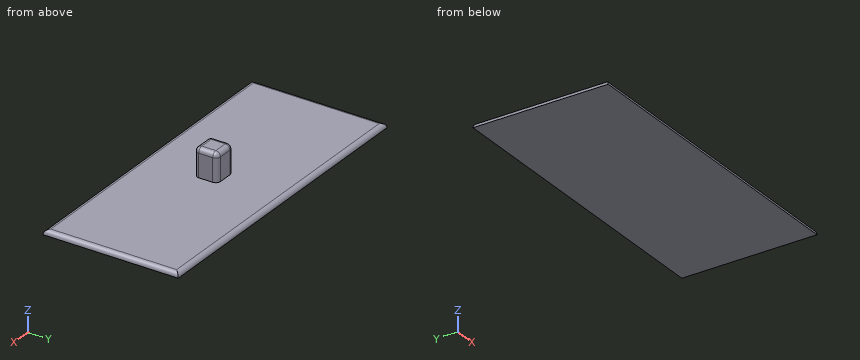
```python
from build123d import *

# Parameters (mm, degrees)
F0_W     = 170.18
F0_H     = 73.66
F1_DEPTH = 2.54
F2_W     = 12.7
F2_H     = 12.7
F3_DEPTH = 15.24
F4_R     = 2.53999


# Not quite as in the source:
# - a fillet or chamfer is up to 0.001 mm smaller than in the source, because OpenCascade refuses the exact size


with BuildPart() as f1:
    # F0 (on Top) → F1 (new body)
    with BuildSketch(Plane.XY):
        with Locations((1.0795005364, 0)):
            Rectangle(F0_W, F0_H)
    extrude(amount=F1_DEPTH)

    # F2 (on face) → F3 (join)
    with BuildSketch(Plane.XY.offset(2.54)):
        with Locations((0, -1.5238544315)):
            Rectangle(F2_W, F2_H)
    extrude(amount=F3_DEPTH)

    # F4 (radius 2.54 in the source; OpenCascade refuses exactly that, so slightly less here)
    f4_edges = [f1.edges().sort_by_distance(p)[0] for p in [
        (0, -7.873854, 17.78),
        (-6.35, -1.523854, 17.78),
        (0, 4.826146, 17.78),
        (6.35, -1.523854, 17.78),
        (-6.35, -7.873854, 10.16),
        (6.35, -7.873854, 10.16),
        (6.35, 4.826146, 10.16),
        (-6.35, 4.826146, 10.16),
        (1.079501, -36.83, 2.54),
        (86.169501, 0, 2.54),
        (1.079501, 36.83, 2.54),
        (-84.010499, 0, 2.54),
    ]]
    fillet(f4_edges, radius=F4_R)


solid = f1.part
```
Can you work these out from the model? Positions are in its coordinate system, mm. Coordinates: 2 decimals unless noted, no trailing zeros. Loops run counter-clockwise (first coordinate to the right, second up) from the corner with the lowest first, then second, coordinate; pieces in that order, holes last.
1) Imagine slicing it at A-A on z = 11.5. List the corners of the cut face in (x, y) for me, plus the area to 3 significant figures.
2) I need wall thicknesses on probe 1 along Z at (x, y) = (-67.5, -3); probe 2 along X at (y, z) = (-6.5, 15.75); probe 3 along X at (y, z) = (1, 15.5). Which ranges of each line are inside material? Lowest first, please.
3) For pin 1 (4 mm diameter, centred on y = -3, z = 10, fed in from -X); pin 2 (2.5 mm diameter, centred on x = 1.5, z = 10.5, fed in from +Y); pin 3 (2.5 mm diameter, centred on x = -0.5, z = 6.5, fed in from -Y); pin 4 (3 mm diameter, centred on x = -41.5, z = 5.5, fed in from +Y), each with a flat end and sliding along its axis, tell me the tip position at first contact or that it passes through.
Completed:
1. outline: (-6.35, -5.33) arc R2.54 ccw to (-3.81, -7.87) - (3.81, -7.87) arc R2.54 ccw to (6.35, -5.33) - (6.35, 2.29) arc R2.54 ccw to (3.81, 4.83) - (-3.81, 4.83) arc R2.54 ccw to (-6.35, 2.29) - close
1. area: 156 mm2
2. probe 1: z = 0 to 2.54
2. probe 2: x = -6.01 to 6.01
2. probe 3: x = -6.34 to 6.34
3. pin 1: stops at x = -6.35
3. pin 2: stops at y = 4.83
3. pin 3: stops at y = -7.87
3. pin 4: passes through
